Build history of the part. All positions in model axes, mm. A direction names the side the tool comes from. Give positions to 0.01 mm unless a question says otherwise; leave off trailing zeros. Write each loop counter-clockwise with the first axis right and the second up, starting at its lowest first coordinate (ties: lowest second). Pieces come first, ordered by that corner, then holes. Notation, with made-up numbers: (-29, 58) - (7, 58) arc R15 cw to (7, 62) - close; hole circle Ø9 at (20, 35). An arc over 180 degrees is marked (long way). Use one line per item in the form item = value. Start each with the question number.
from build123d import *

# Parameters (mm, degrees)
F0_W     = 25.5778
F0_H     = 6.4389
F1_DEPTH = 6.35


with BuildPart() as f1:
    # F0 (on Front) → F1 (new body)
    with BuildSketch(Plane.XZ):
        Polygon((0, 25.4889), (0, 0), (25.3111, 0), (50.8889, 0), (76.1111, 0), (101.6889, 0), (126.9111, 0), (152.4889, 0), (177.8, 0), (177.8, 25.4889), (171.5389, 25.4889), (171.5389, 50.7111), (177.8, 50.7111), (177.8, 76.2889), (171.5389, 76.2889), (171.5389, 101.5111), (177.8, 101.5111), (177.8, 127), (0, 127), (0, 101.5111), (6.2611, 101.5111), (6.2611, 76.2889), (0, 76.2889), (0, 50.7111), (6.2611, 50.7111), (6.2611, 25.4889), align=None)
        with Locations((38.1, -3.21945)):
            Rectangle(F0_W, F0_H)
        with Locations((88.9, -3.21945)):
            Rectangle(F0_W, F0_H)
        with Locations((139.7, -3.21945)):
            Rectangle(F0_W, F0_H)
    extrude(amount=F1_DEPTH)


solid = f1.part
(1) Cut at C-C, the plane x = 159. Give the cut face in (y, z), then the cut area to 3 significant figures.
(2) Cut at B-B, the plane z = 86. Give the cut face in (x, y), then the cut area to 3 significant figures.
(3) Which spindle directions (+Z, -Z, +X, -X, +Y, -Y) get a long thin tool onto all of the face, cutting with end or side? Do faces 4 (the flat face through (3, -3, 76.289)), 5 (the flat face through (114, -3, 0)), 6 (the flat face through (25.311, -3, -3)), 7 (the flat face through (171.539, -3, 89)). Say none if no direction does.
(4) Pin check, flat tip, straight feed: pin 1 Ø3 at (x, y) = (3.5, -4.5) entering from -Z. Stop position of the tip, or through.
(5) Wall check: line 1 (Z direction, x = 69.5, y = -3.75); line 2 (X direction, y = -2.75, z = 39). Give the ranges that are in metal, low to high. Write a range as from..to.
(6) Two-plate mould, pull along Z, no slides. Class faces 1 (the flat face through (76.111, -3, -3)), 2 (the flat face through (140, -3, -6.439)), 3 (the flat face through (6.261, -3, 38)): +Z half, -Z half, draft (parallel to the pull), parting line (faces both ways), or undercut.
Solution:
q1.outline = (-6.35, 0) - (0, 0) - (0, 127) - (-6.35, 127) - close
q1.area = 806 mm2
q2.outline = (6.26, -6.35) - (171.54, -6.35) - (171.54, 0) - (6.26, 0) - close
q2.area = 1,050 mm2
q3.face_4 = -X, +Y, -Y
q3.face_5 = -Z, +Y, -Y
q3.face_6 = -Z, -X, +Y, -Y
q3.face_7 = +X, +Y, -Y
q4.pin_1 = 0
q5.line_1 = 0..127
q5.line_2 = 6.26..171.54
q6.face_1 = draft
q6.face_2 = -Z half
q6.face_3 = undercut
